Can you work these out from the model? Positions are in its coordinate system, mm. Coordinates: 2 decimals unless noted, no trailing zeros. Order: outer loops, then holes, each group sorted by start corner. A loop starts at its lowest first (then second) coordinate and runs counter-clockwise, first axis right, second up. Notation, with made-up numbers: (2.5, 75) -> (34.5, 75) arc R18 cw to (34.5, 83) -> close; hole circle Ø7 at (41, 51). An arc over 180 degrees is marked (long way). Use a Markdown table: item, result. Add a question column.
1. Suppose I cut it at C-C, the plane y = 0. List the corners of the cut face in (x, z) for me, then the cut area to 3 significant figures.
2. Suppose I cut it at A-A, the plane x = -12.7. List the corners of the cut face in (y, z) for me, then the cut area to 3 significant figures.
3. If I drill on line 1 along Y through (x, z) = (-12.7, -3.8); line 2 along X through (y, z) = (1.75, -1); line 3 along Y through (x, z) = (-13, -1.2), over which ranges is the centre line in solid material (lowest first)? Write a range as from..to.
4. Suppose I cut it at B-B, the plane z = -0.5. List the corners of the cut face in (x, y) for me, then the cut area to 3 significant figures.
5. We'd pull the mould along X, two halves only. Please class faces 1 (the cylindrical face through (-15.29, -1.986, -2.348)), 2 (the flat face through (0, 0, -4.762)), 3 (the flat face through (-25.4, 0, -2)): pulls with the +X half, pulls with the -X half, needs draft (parallel to the pull), parting line crosses it, or undercut.
```python
from build123d import *

# Parameters (mm, degrees)
SKETCH1_W      = 50.8
SKETCH1_H      = 22.225
SKETCH1_R      = 3.2639
EXTRUDE1_DEPTH = 4.7625


with BuildPart() as part:
    # Sketch1 → Extrude1 (new body)
    with BuildSketch(Plane.XY):
        Rectangle(SKETCH1_W, SKETCH1_H)
        with Locations((12.7, 0)):
            Circle(SKETCH1_R, mode=Mode.SUBTRACT)
        with Locations((-12.7, 0)):
            Circle(SKETCH1_R, mode=Mode.SUBTRACT)
    extrude(amount=-EXTRUDE1_DEPTH)


solid = part.part
```
Worked out:
| question | item | result |
|---|---|---|
| 1 | outline | (-25.4, -4.76) -> (-15.96, -4.76) -> (-15.96, 0) -> (-25.4, 0) -> close; (-9.44, -4.76) -> (9.44, -4.76) -> (9.44, 0) -> (-9.44, 0) -> close; (15.96, -4.76) -> (25.4, -4.76) -> (25.4, 0) -> (15.96, 0) -> close |
| 1 | area | 180 mm² |
| 2 | outline | (-11.11, -4.76) -> (-3.26, -4.76) -> (-3.26, 0) -> (-11.11, 0) -> close; (3.26, -4.76) -> (11.11, -4.76) -> (11.11, 0) -> (3.26, 0) -> close |
| 2 | area | 74.8 mm² |
| 3 | line 1 | y = -11.11..-3.26, 3.26..11.11 |
| 3 | line 2 | x = -25.4..-15.46, -9.94..9.94, 15.46..25.4 |
| 3 | line 3 | y = -11.11..-3.25, 3.25..11.11 |
| 4 | outline | (-25.4, -11.11) -> (25.4, -11.11) -> (25.4, 11.11) -> (-25.4, 11.11) -> close; hole circle Ø6.53 at (-12.7, 0); hole circle Ø6.53 at (12.7, 0) |
| 4 | area | 1,060 mm² |
| 5 | face 1 | undercut |
| 5 | face 2 | needs draft |
| 5 | face 3 | pulls with the -X half |
